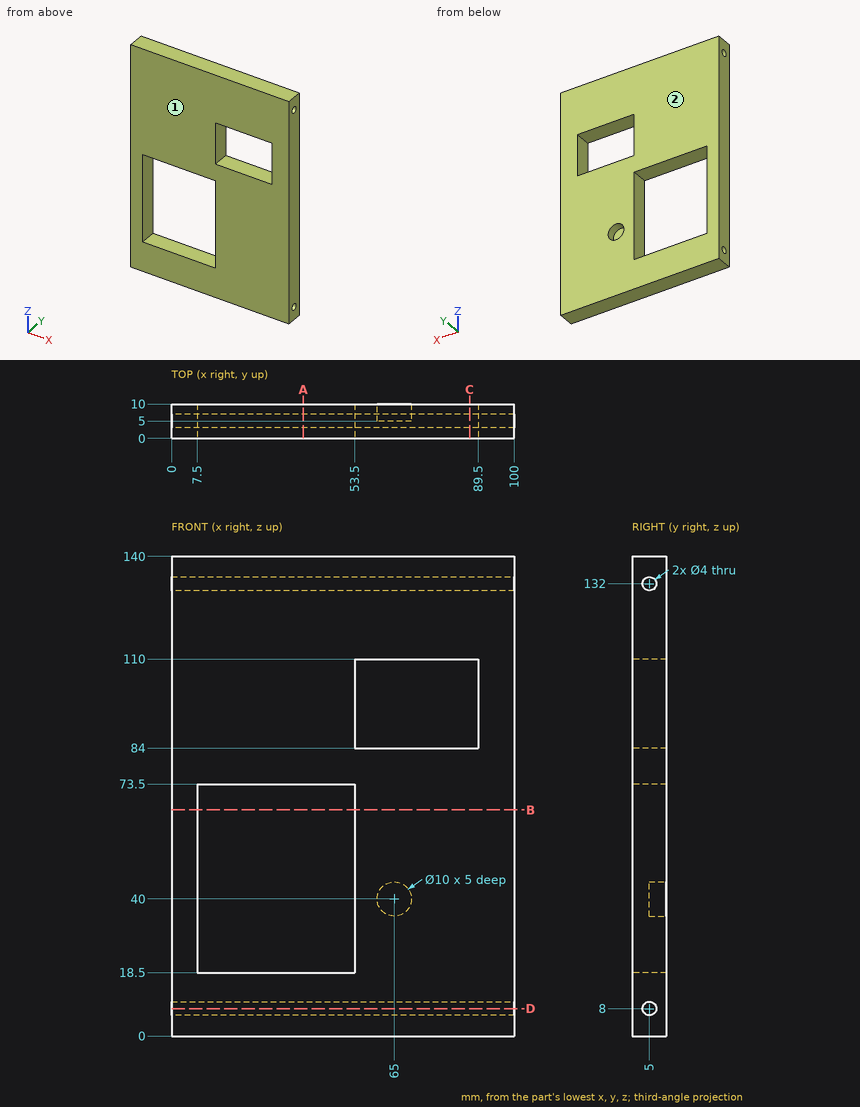
Study the drawing (mm; zero at the part's minimum x, y, z) and answer. Round coordinates to 2 decimals unless told otherwise and drop trailing zeros. Loops run counter-clockwise (first coordinate to the right, second up) from the corner with the lowest first, then second, coordinate; pieces in that order, holes last. Notation, with made-up numbers: (55, 56.5) -> (107, 56.5) arc R35 ccw to (107, 94.5) -> close; hole circle Ø10 at (29, 61). An arc over 180 degrees is marked (long way). One line per item, written item: value.
1) Flat-ended cylindrical pins translate along their axes: P1, Ø5, axis at x = 66, z = 42.5, coming from the +Y side; P2, Ø6, axis at x = 65, z = 40, coming from the +Y side. Find the tip coordinate at first contact, or state that the pin passes through.
Answer list:
P1: stops at y = 10
P2: stops at y = 5
2) A cutting plane is placed at B-B (z = 66). Determine the outline of the cut face in (x, y).
Answer list:
outline: (0, 0) -> (7.5, 0) -> (7.5, 10) -> (0, 10) -> close; (53.5, 0) -> (100, 0) -> (100, 10) -> (53.5, 10) -> close
3) The mould has two halves that part along Y. Classify the marked faces 1 and 2: pulls with the +Y half, pulls with the -Y half, needs draft (parallel to the pull), parting line crosses it, or undercut.
Answer list:
face 1: pulls with the -Y half
face 2: pulls with the +Y half
4) Consider L1, parallel to X at y = 7.5, z = 40; L2, parallel to Z at x = 65, y = 7.8; L3, parallel to X at y = 1.25, z = 90. Determine where each line is inside the solid, lowest interval first. Write a range as [from, to].
Answer list:
L1: x = [0, 7.5], [53.5, 60], [70, 100]
L2: z = [0, 35], [45, 84], [110, 140]
L3: x = [0, 53.5], [89.5, 100]
5) A cutting plane is placed at A-A (x = 38.5). Determine the outline of the cut face in (y, z), and give its area (3 significant figures).
Answer list:
outline: (0, 0) -> (10, 0) -> (10, 18.5) -> (0, 18.5) -> close; (0, 73.5) -> (10, 73.5) -> (10, 140) -> (0, 140) -> close; hole circle Ø4 at (5, 8); hole circle Ø4 at (5, 132)
area: 825 mm²
6) A cutting plane is placed at C-C (x = 87). Determine the outline of the cut face in (y, z).
Answer list:
outline: (0, 0) -> (10, 0) -> (10, 84) -> (0, 84) -> close; (0, 110) -> (10, 110) -> (10, 140) -> (0, 140) -> close; hole circle Ø4 at (5, 8); hole circle Ø4 at (5, 132)
7) A cutting plane is placed at D-D (z = 8). Determine the outline of the cut face in (x, y), and give its area (3 significant figures).
Answer list:
outline: (0, 0) -> (100, 0) -> (100, 3) -> (0, 3) -> close; (0, 7) -> (100, 7) -> (100, 10) -> (0, 10) -> close
area: 600 mm²
